Autodesk Inventor part; units mm, degrees
ref_plane "YZ Plane" through (0, 0, 0) normal (1, 0, 0) x (0, 1, 0)
ref_plane "XZ Plane" through (0, 0, 0) normal (0, 1, 0) x (-1, 0, 0)
ref_plane "XY Plane" through (0, 0, 0) normal (0, 0, 1) x (1, 0, 0)
sketch "Sketch1" plane through (0, 0, 0) normal (1, 0, 0) x (0, 1, 0)
  line L0 (0, 0) -> (0, -30)
  line L1 (0, -30) -> (27, -30)
  line L2 (27, -30) -> (27, 0)
  line L3 (27, 0) -> (18, 0)
  line L4 (18, 0) -> (18, 30)
  line L5 (18, 30) -> (9, 30)
  line L6 (9, 30) -> (9, 0)
  line L7 (9, 0) -> (0, 0)
  dimension "d0" = 30
  dimension "d1" = 27
  dimension "d3" = 9
  dimension "d4" = 9
  dimension "d5" = 30
extrude "Extrusion1" add sketch "Sketch1" along normal mid plane 24
fillet "Fillet1" radius 12 1 edges at (12, 13.5, 30)
fillet "Fillet2" radius 12 1 edges at (-12, 13.5, 30)
sketch "Sketch2" plane through (-12, 18, 0) normal (0, 1, 0) x (1, 0, 0)
  circle A0 centre (12, -18) radius 6
  line L0 (0, 0) -> (24, 0)
  line L1 (0, 30) -> (24, 30)
  point P0 (12, 0)
  dimension "d10" = 12
  dimension "d11" = 18
sketch "Sketch3" plane through (-12, 27, 0) normal (0, 1, 0) x (1, 0, 0)
  line L0 (0, 30) -> (24, 30)
  line L1 (8, 30) -> (8, 10.1515)
  line L2 (8, 10.1515) -> (16, 10.1515)
  line L3 (16, 10.1515) -> (16, 30)
  line L4 (24, 30) -> (24, 0)
  line L5 (8, 30) -> (16, 30)
  point P0 (12, 0)
  dimension "d12" = 8
  dimension "d13" = 8
extrude "Extrusion2" cut sketch "Sketch2" against normal through all
extrude "Extrusion3" cut sketch "Sketch3" against normal through all
Input: part model. Units: mm. Frame: model coordinates. A direction names the side the tool comes from. Give positions to 0.01 mm unless a question says otherwise; leave off trailing zeros. Write each loop counter-clockwise with the first axis right and the second up, starting at its lowest first coordinate (ties: lowest second). Pieces come first, ordered by that corner, then holes.
Q1. Section B-B, the plane x = 5.25. Output: boundary loops of the cut face in (y, z), plus the area to 3 significant figures.
Q2. Material intervals for probe 1 along X at (y, z) = (15.25, 18); probe 2 along Z at (x, y) = (0, 16); probe 3 along X at (y, z) = (6.5, -19.5), sorted ascending.
Q3. Section A-A, the plane z = -19. Output: boundary loops of the cut face in (x, y), plus the area to 3 significant figures.
Q4. First-contact query: P1, Ø7, axis at x = 4, z = 20, coming from the +Y side; P2, Ø4.5, axis at x = -5.5, y = 5.5, coming from the +Z side; P3, Ø8, axis at x = 3.5, y = 9.5, coming from the -Z side. Flat tips, straight axial feed; report the tip coordinate or a pass-through.
Q5. Section C-C, the plane y = 24.75. Output: boundary loops of the cut face in (x, z).
Q6. Set-up query: faces 4 (the face through (0, 23, 0)), 5 (the face through (0, 14, -10.152)), 6 (the face through (0, 5, 0)). Return all of +Z, -Z, +X, -X, +Y, -Y with unobstructed straight access to the full face (end or side cutting, diameter ignored); none if empty.
Q7. Pull-direction query (X, two-part tool) for faces 1 (the face through (-12, 13, -11)), 2 (the face through (-4, 14, -20)), 3 (the face through (8.58, 13.44, 26.39)); classes: pulls with the +X half, pulls with the -X half, needs draft (parallel to the pull), parting line crosses it, or undercut.
Q8. Section D-D, the plane x = 2. Output: boundary loops of the cut face in (y, z), plus the area to 3 significant figures.
Filled in:
1. outline: (0, -30) - (27, -30) - (27, 0) - (18, 0) - (18, 15.1) - (9, 15.1) - (9, 0) - (0, 0) - close; (9, 20.9) - (18, 20.9) - (18, 28.79) - (9, 28.79) - close
1. area: 1,020 mm2
2. probe 1: x = -12 to -6, 6 to 12
2. probe 2: z = -10.15 to 12, 24 to 30
2. probe 3: x = -12 to -4, 4 to 12
3. outline: (-12, 0) - (-4, 0) - (-4, 27) - (-12, 27) - close; (4, 0) - (12, 0) - (12, 27) - (4, 27) - close
3. area: 432 mm2
4. P1: stops at y = 18
4. P2: stops at z = 0
4. P3: stops at z = -30
5. outline: (-12, -30) - (-4, -30) - (-4, -10.15) - (4, -10.15) - (4, -30) - (12, -30) - (12, 0) - (-12, 0) - close
6. face 4: +Z, +X, -X, +Y
6. face 5: -Z, +Y, -Y
6. face 6: +Z, +X, -X, -Y
7. face 1: pulls with the -X half
7. face 2: undercut
7. face 3: pulls with the +X half
8. outline: (0, -10.15) - (27, -10.15) - (27, 0) - (18, 0) - (18, 12.34) - (9, 12.34) - (9, 0) - (0, 0) - close; (9, 23.66) - (18, 23.66) - (18, 29.83) - (9, 29.83) - close
8. area: 441 mm2
